The model under review builds one solid part; all positions refer to its coordinate system, in mm. Coordinates: 2 decimals unless noted, no trailing zeros. Write each loop counter-clockwise with the first axis right and the second up, starting at its lowest first coordinate (ties: lowest second). Pieces come first, ordered by that corner, then holes. Notation, with made-up numbers: (75, 50) - (83, 50) arc R13 ccw to (83, 64) - close; hole circle Ø6 at (-36, 4.5). An arc over 180 degrees is marked (long way). Use one line per item in the form item = value. Start each with the question number.
```python
from build123d import *

# Parameters (mm, degrees)
F0_R     = 38.0365
F1_DEPTH = 254
F2_R     = 27.5008894084
F3_DEPTH = 25.4
F4_R     = 25.39999


# Not quite as in the source:
# - a fillet or chamfer is up to 0.001 mm smaller than in the source, because OpenCascade refuses the exact size


with BuildPart() as f1:
    # F0 (on Right) → F1 (new body)
    with BuildSketch(Plane.YZ):
        Circle(F0_R)
    extrude(amount=F1_DEPTH)

    # F2 (on face) → F3 (cut)
    with BuildSketch(Plane.YZ.offset(254)):
        Circle(F2_R)
    extrude(amount=-F3_DEPTH, mode=Mode.SUBTRACT)

    # F4 (radius 25.4 in the source; OpenCascade refuses exactly that, so slightly less here)
    f4_edges = [f1.edges().sort_by_distance(p)[0] for p in [
        (228.6, -27.500889, 0),
    ]]
    fillet(f4_edges, radius=F4_R)


solid = f1.part
```
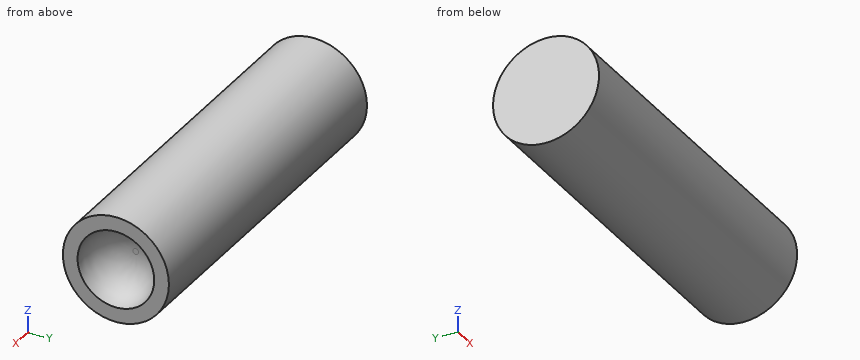
1. For L1, parallel to Z at x = 240, y = -17; L2, parallel to X at y = 12, z = 4.5; L3, parallel to Y at x = 209, z = 12.5, list the stretches that pass through material, from the lowest coordinate up.
2. Take a section at B-B (y = -30). State the section outline as (x, z) points, plus the area to 3 significant figures.
3. For P1, Ø1.5, axis at x = 124, y = 19.5, coming from the +Z side; P2, Ø6, axis at x = 66.5, z = 19.5, coming from the -Y side; P3, Ø1, axis at x = 194, y = 19, coming from the -Z side, all flat-tipped, find the tip position at first contact; note any pin that passes through.
4. Take a section at A-A (x = 203). State the section outline as (y, z) points.
Returned:
q1.L1 = -34.03 to -15.93, 15.93 to 34.03
q1.L2 = 0 to 230.97
q1.L3 = -35.92 to 35.92
q2.outline = (0, -23.38) - (254, -23.38) - (254, 23.38) - (0, 23.38) - close
q2.area = 11,900 mm²
q3.P1 = 33.09
q3.P2 = -34.27
q3.P3 = -33.23
q4.outline = circle Ø76.07 at (0, 0)
